```python
from build123d import *

# Parameters (mm, degrees)
F1_DEPTH = 10
F0_R     = 9
F0_R_2   = 8.5
F0_W     = 35.6
F0_H     = 3
F2_DEPTH = 2.5
F0_W_2   = 39
F0_W_3   = 20.3
F3_DEPTH = 5
F5_DEPTH = 10
F7_DEPTH = 43


with BuildPart() as f1:
    # F0 (on Top) → F1 (new body)
    with BuildSketch(Plane.XY):
        Polygon((-60, 5), (-60, -5), (-35.75, -5), (44.2, -5), (60, -5), (60, 5), (58.5, 5), (45.2, 5), (44.2, 5), (30.9, 5), (29.9, 5), (16.6, 5), (15.6, 5), (2.3, 5), (1.3, 5), (-12, 5), (-13, 5), (-27.5, 5), (-28.5, 5), (-43, 5), (-44, 5), (-58.5, 5), align=None)
    extrude(amount=F1_DEPTH)

    # F0 (on Top) → F2 (join)
    with BuildSketch(Plane.XY):
        with BuildLine():
            Line((44.2, -5), (-35.75, -5))
            ThreePointArc((-35.75, -5), (-0.3225250219, -43.4311769232), (-8.85, -95))
            Line((-8.85, -95), (26.75, -95))
            Line((26.75, -95), (26.75, -98))
            ThreePointArc((26.75, -98), (38.9235283255, -86.984743063), (54.85, -83))
            Line((54.85, -83), (34.55, -83))
            Line((34.55, -83), (34.55, -80))
            Line((34.55, -80), (54.85, -80))
            ThreePointArc((54.85, -80), (16.9738118998, -47.1222687102), (44.2, -5))
        make_face()
        with Locations((15.8479269594, -78.1992301345)):
            Circle(F0_R, mode=Mode.SUBTRACT)
        with Locations((6.0314284638, -16.3851659745)):
            Circle(F0_R_2, mode=Mode.SUBTRACT)
        with BuildLine():
            Line((-8.85, -98), (-8.85, -95))
            ThreePointArc((-8.85, -95), (-29.1337234425, -112.9126092907), (-55.25, -120))
            Line((-55.25, -120), (-16.25, -120))
            Line((-16.25, -120), (-16.25, -123))
            ThreePointArc((-16.25, -123), (1.8803397691, -104.7041844029), (26.75, -98))
            Line((26.75, -98), (-8.85, -98))
        make_face()
        with Locations((8.95, -96.5)):
            Rectangle(F0_W, F0_H)
    extrude(amount=F2_DEPTH)

    # F0 (on Top) → F3 (join)
    with BuildSketch(Plane.XY):
        with Locations((-35.75, -121.5)):
            Rectangle(F0_W_2, F0_H)
        with Locations((8.95, -96.5)):
            Rectangle(F0_W, F0_H)
        with Locations((44.7, -81.5)):
            Rectangle(F0_W_3, F0_H)
    extrude(amount=F3_DEPTH)

    # F4 (on face) → F5 (cut, through all)
    with BuildSketch(Plane(origin=(0, 5, 0), x_dir=(-1, 0, 0), z_dir=(0, 1, 0))):
        with BuildLine():
            Line((-45.2016919446, 10), (-58.4983080554, 10))
            ThreePointArc((-58.4983080554, 10), (-51.85, 3.5), (-45.2016919446, 10))
        make_face()
        with BuildLine():
            Line((-30.9016919446, 10), (-44.1983080554, 10))
            ThreePointArc((-44.1983080554, 10), (-37.55, 3.5), (-30.9016919446, 10))
        make_face()
        with BuildLine():
            Line((-16.6016919446, 10), (-29.8983080554, 10))
            ThreePointArc((-29.8983080554, 10), (-23.25, 3.5), (-16.6016919446, 10))
        make_face()
        with BuildLine():
            ThreePointArc((-15.5983080554, 10), (-8.95, 3.5), (-2.3016919446, 10))
            Line((-2.3016919446, 10), (-15.5983080554, 10))
        make_face()
        with BuildLine():
            ThreePointArc((-1.2983080554, 10), (5.35, 3.5), (11.9983080554, 10))
            Line((11.9983080554, 10), (-1.2983080554, 10))
        make_face()
        with BuildLine():
            ThreePointArc((13.0043116269, 10), (20.25, 3), (27.4956883731, 10))
            Line((27.4956883731, 10), (13.0043116269, 10))
        make_face()
        with BuildLine():
            ThreePointArc((28.5043116269, 10), (35.75, 3), (42.9956883731, 10))
            Line((42.9956883731, 10), (28.5043116269, 10))
        make_face()
        with BuildLine():
            ThreePointArc((44.0043116269, 10), (51.25, 3), (58.4956883731, 10))
            Line((58.4956883731, 10), (44.0043116269, 10))
        make_face()
    extrude(amount=-F5_DEPTH, mode=Mode.SUBTRACT)

    # F6 (on face) → F7 (cut, through all)
    with BuildSketch(Plane.XZ.offset(123)):
        with BuildLine():
            Line((-49.159545504, 5), (-53.340454496, 5))
            ThreePointArc((-53.340454496, 5), (-51.25, 3.1), (-49.159545504, 5))
        make_face()
        with BuildLine():
            Line((-33.659545504, 5), (-37.840454496, 5))
            ThreePointArc((-37.840454496, 5), (-35.75, 3.1), (-33.659545504, 5))
        make_face()
        with BuildLine():
            ThreePointArc((-22.340454496, 5), (-20.25, 3.1), (-18.159545504, 5))
            Line((-18.159545504, 5), (-22.340454496, 5))
        make_face()
        with BuildLine():
            Line((-4.3107695155, 5), (-6.3892304845, 5))
            ThreePointArc((-6.3892304845, 5), (-5.35, 4.1), (-4.3107695155, 5))
        make_face()
        with BuildLine():
            ThreePointArc((7.9107695155, 5), (8.95, 4.1), (9.9892304845, 5))
            Line((9.9892304845, 5), (7.9107695155, 5))
        make_face()
        with BuildLine():
            ThreePointArc((22.2107695155, 5), (23.25, 4.1), (24.2892304845, 5))
            Line((24.2892304845, 5), (22.2107695155, 5))
        make_face()
        with BuildLine():
            Line((38.5892304845, 5), (36.5107695155, 5))
            ThreePointArc((36.5107695155, 5), (37.55, 4.1), (38.5892304845, 5))
        make_face()
        with BuildLine():
            Line((52.8892304845, 5), (50.8107695155, 5))
            ThreePointArc((50.8107695155, 5), (51.85, 4.1), (52.8892304845, 5))
        make_face()
    extrude(amount=-F7_DEPTH, mode=Mode.SUBTRACT)


solid = f1.part
```
Can you work these out from the model? Positions are in its coordinate system, mm. A direction names the side the tool comes from. Coordinates: 2 decimals unless noted, no trailing zeros. Write each loop counter-clockwise with the first axis right and the second up, starting at its lowest first coordinate (ties: lowest second). Pieces come first, ordered by that corner, then holes. Notation, with made-up numbers: M 50.25,-38 L 101.25,-38 A22 ccw 101.25,-31 Z; hole C -7.75,-21.5 d3. An arc over 180 degrees is marked long. Write item = value, one per line. Start each with the question number.
Q1. On a 3-axis mill with a long thin cutter (end or side, diameter ignored), from which of +Z, -Z, +X, -X, +Y, -Y can I reach the whole of each face in a straight line? I mean faces 1 (the face through (-60, 0, 5)), 2 (the face through (-5.2, 0.1, 3.5)), 3 (the face through (-28, -121, 5)). Say none if no direction works.
Q2. Thinking about a two-plate mould opening in X: for faces 4 (the face through (-44, -121, 5)), 5 (the face through (9.1, 0.1, 3.5)), 6 (the face through (1.566, -104.889, 1.232)), which applies, released by +X, released by -X, zero draft, split by the parting line, or undercut?
Q3. If we section it at C-C, the plane x = -51.25: Write out the boundary of the cut face in (y, z), then the cut area to 3 significant figures.
Q4. I'm going to push flat-ended pins straight in: pin 1 (2 mm diameter, centred on x = 25, y = -97, fed in from +Z); pin 2 (0.8 mm diameter, centred on y = -81.5, z = 4, fed in from -X); pin 3 (22 mm diameter, centred on x = 6.03, y = -16.39, fed in from +Z); pin 4 (1.5 mm diameter, centred on x = 0.5, y = -57, fed in from -Z) (1 decimal). Where does each tip first touch, or does it pass through?
Q5. If we section it at B-B, the plane y = -9.5: Write out the boundary of the cut face in (x, z).
Q6. If we section it at D-D, the plane z = 8: State how many separate pieces and enclosed holes the cut face has, then the cut area to 3 significant figures.
Q7. If I drill on L1, parallel to Y at x = 10.5, z = 3.5; L2, parallel to Y at x = -41.5, z = 4.25; L3, parallel to Z at x = 13, y = -66, over which ranges is the centre line in solid material (lowest first)? Write a range as [from, to].
Q8. If we section it at A-A, the plane x = 33: Write out the boundary of the cut face in (y, z).
Check sheet entries:
q1.face_1 = +Z, -Z, -X, +Y, -Y
q1.face_2 = +Z, +Y
q1.face_3 = +Z, +X, -X, -Y
q2.face_4 = zero draft
q2.face_5 = undercut
q2.face_6 = released by +X
q3.outline = M -123,0 L -119.72,0 L -119.72,2.5 L -120,2.5 L -120,3.1 L -123,3.1 Z; M -5,0 L 5,0 L 5,3 L -5,3 Z
q3.area = 40.0 mm²
q4.pin_1 = 5
q4.pin_2 = 34.55
q4.pin_3 = 2.5
q4.pin_4 = through
q5.outline = M -26.61,0 L 1.05,0 L 1.05,2.5 L -26.61,2.5 Z; M 11.02,0 L 34.26,0 L 34.26,2.5 L 11.02,2.5 Z
q6.separate_pieces = 9
q6.enclosed_holes = 0
q6.area = 157 mm²
q7.L1 = [-98, -95], [-5, 5]
q7.L2 = [-123, -120], [-5, 5]
q7.L3 = [0, 2.5]
q8.outline = M -91.01,0 L -73.15,0 L -73.15,2.5 L -91.01,2.5 Z; M -10.34,0 L 5,0 L 5,5.3 L -5,5.3 L -5,2.5 L -10.34,2.5 Z
